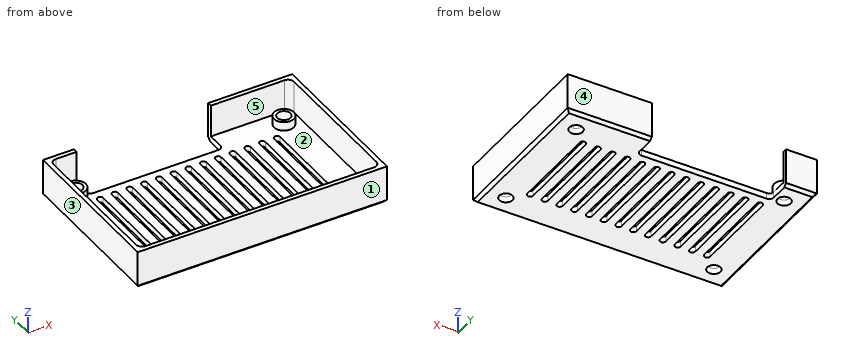
```python
from build123d import *

# Parameters (mm, degrees)
F0_W      = 84.5
F0_H      = 54
F1_DEPTH  = 11
F2_W      = 84.5
F2_H      = 54
F3_DEPTH  = 2
F4_R      = 2.25
F5_DEPTH  = 12.5
F6_R      = 3.35
F6_R_2    = 2.25
F7_DEPTH  = 3
F8_SIZE   = 1
F10_DEPTH = 2


with BuildPart() as f1:
    # F0 (on Top) → F1 (new body)
    with BuildSketch(Plane.XY):
        Rectangle(F0_W, F0_H)
        with BuildLine():
            Line((-40.75, -23.5), (-40.75, 23.5))
            ThreePointArc((-40.75, 23.5), (-40.164214, 24.914214), (-38.75, 25.5))
            Line((-38.75, 25.5), (38.75, 25.5))
            ThreePointArc((38.75, 25.5), (40.164214, 24.914214), (40.75, 23.5))
            Line((40.75, 23.5), (40.75, -23.5))
            ThreePointArc((40.75, -23.5), (40.164214, -24.914214), (38.75, -25.5))
            Line((38.75, -25.5), (-38.75, -25.5))
            ThreePointArc((-38.75, -25.5), (-40.164214, -24.914214), (-40.75, -23.5))
        make_face(mode=Mode.SUBTRACT)
    extrude(amount=F1_DEPTH)

    # F2 (on face) → F3 (join)
    with BuildSketch(Plane(origin=(0, 0, 0), x_dir=(1, 0, 0), z_dir=(0, 0, -1))):
        Rectangle(F2_W, F2_H)
    extrude(amount=F3_DEPTH)

    # F4 (on face) → F5 (cut, symmetric)
    with BuildSketch(Plane.XY):
        with Locations((-35.25, 20)):
            Circle(F4_R)
        with BuildLine():
            ThreePointArc((-31.75, 20), (-31.31066, 18.93934), (-30.25, 18.5))
            Line((-30.25, 18.5), (12.25, 18.5))
            ThreePointArc((12.25, 18.5), (13.31066, 18.93934), (13.75, 20))
            Line((13.75, 20), (13.75, 27))
            Line((13.75, 27), (-31.75, 27))
            Line((-31.75, 27), (-31.75, 20))
        make_face()
        with Locations((-35.25, -20)):
            Circle(F4_R)
        with Locations((35.25, 20)):
            Circle(F4_R)
        with Locations((35.25, -20)):
            Circle(F4_R)
    extrude(amount=F5_DEPTH, both=True, mode=Mode.SUBTRACT)

    # F6 (on face) → F7 (join)
    with BuildSketch(Plane.XY):
        with Locations((-35.25, 20)):
            Circle(F6_R)
        with Locations((-35.25, 20)):
            Circle(F6_R_2, mode=Mode.SUBTRACT)
        with Locations((35.25, 20)):
            Circle(F6_R)
        with Locations((35.25, 20)):
            Circle(F6_R_2, mode=Mode.SUBTRACT)
        with Locations((-35.25, -20)):
            Circle(F6_R)
        with Locations((-35.25, -20)):
            Circle(F6_R_2, mode=Mode.SUBTRACT)
        with Locations((35.25, -20)):
            Circle(F6_R)
        with Locations((35.25, -20)):
            Circle(F6_R_2, mode=Mode.SUBTRACT)
    extrude(amount=F7_DEPTH)

    # F8
    f8_edges = [f1.edges().sort_by_distance(p)[0] for p in [
        (-42.25, 0, -2),
        (-37, 27, -2),
        (28, 27, -2),
        (0, -27, -2),
        (42.25, 0, -2),
    ]]
    chamfer(f8_edges, length=F8_SIZE)

    # F9 (on face) → F10 (cut, through all)
    with BuildSketch(Plane.XY):
        with BuildLine():
            ThreePointArc((1, 15), (0, 16), (-1, 15))
            Line((-1, 15), (-1, -15))
            ThreePointArc((-1, -15), (0, -16), (1, -15))
            Line((1, -15), (1, 15))
        make_face()
        with BuildLine():
            Line((6, -15), (6, 15))
            ThreePointArc((6, 15), (5, 16), (4, 15))
            Line((4, 15), (4, -15))
            ThreePointArc((4, -15), (5, -16), (6, -15))
        make_face()
        with BuildLine():
            Line((11, -15), (11, 15))
            ThreePointArc((11, 15), (10, 16), (9, 15))
            Line((9, 15), (9, -15))
            ThreePointArc((9, -15), (10, -16), (11, -15))
        make_face()
        with BuildLine():
            Line((16, -15), (16, 15))
            ThreePointArc((16, 15), (15, 16), (14, 15))
            Line((14, 15), (14, -15))
            ThreePointArc((14, -15), (15, -16), (16, -15))
        make_face()
        with BuildLine():
            Line((21, -15), (21, 15))
            ThreePointArc((21, 15), (20, 16), (19, 15))
            Line((19, 15), (19, -15))
            ThreePointArc((19, -15), (20, -16), (21, -15))
        make_face()
        with BuildLine():
            Line((26, -15), (26, 15))
            ThreePointArc((26, 15), (25, 16), (24, 15))
            Line((24, 15), (24, -15))
            ThreePointArc((24, -15), (25, -16), (26, -15))
        make_face()
        with BuildLine():
            Line((-4, -15), (-4, 15))
            ThreePointArc((-4, 15), (-5, 16), (-6, 15))
            Line((-6, 15), (-6, -15))
            ThreePointArc((-6, -15), (-5, -16), (-4, -15))
        make_face()
        with BuildLine():
            Line((-9, -15), (-9, 15))
            ThreePointArc((-9, 15), (-10, 16), (-11, 15))
            Line((-11, 15), (-11, -15))
            ThreePointArc((-11, -15), (-10, -16), (-9, -15))
        make_face()
        with BuildLine():
            Line((-14, -15), (-14, 15))
            ThreePointArc((-14, 15), (-15, 16), (-16, 15))
            Line((-16, 15), (-16, -15))
            ThreePointArc((-16, -15), (-15, -16), (-14, -15))
        make_face()
        with BuildLine():
            Line((-19, -15), (-19, 15))
            ThreePointArc((-19, 15), (-20, 16), (-21, 15))
            Line((-21, 15), (-21, -15))
            ThreePointArc((-21, -15), (-20, -16), (-19, -15))
        make_face()
        with BuildLine():
            Line((-24, -15), (-24, 15))
            ThreePointArc((-24, 15), (-25, 16), (-26, 15))
            Line((-26, 15), (-26, -15))
            ThreePointArc((-26, -15), (-25, -16), (-24, -15))
        make_face()
        with BuildLine():
            Line((-29, -15), (-29, 15))
            ThreePointArc((-29, 15), (-30, 16), (-31, 15))
            Line((-31, 15), (-31, -15))
            ThreePointArc((-31, -15), (-30, -16), (-29, -15))
        make_face()
        with BuildLine():
            Line((31, -15), (31, 15))
            ThreePointArc((31, 15), (30, 16), (29, 15))
            Line((29, 15), (29, -15))
            ThreePointArc((29, -15), (30, -16), (31, -15))
        make_face()
    extrude(amount=-F10_DEPTH, mode=Mode.SUBTRACT)


solid = f1.part
```
For this review, take the finished solid that the model builds, in its own axes (mm). Face numbers are marked on the shaded views. A direction names the side the tool comes from. Coordinates: 2 decimals unless noted, no trailing zeros. Write each loop counter-clockwise with the first axis right and the second up, starting at its lowest first coordinate (ties: lowest second). Pieces come first, ordered by that corner, then holes. Notation, with made-up numbers: (5, -28) - (58, -28) arc R24 cw to (58, -6) - close; hole circle Ø9 at (-28, 86.5). An arc over 180 degrees is marked (long way). Answer in a Markdown table with one row per item. Add a question column.
Q1. Tool access review of the marked faces 4 and 5: name each direction out of +Z, -Z, +X, -X, +Y, -Y from which nothing blocks a thin tool from reaching the whole face with its end or side.
Q2. For probe 1 along Y at (x, z) = (-35.25, -0.8); probe 2 along Y at (x, z) = (-35.25, 0.9); probe 3 along Y at (x, z) = (35.25, -1.2), list the stretches that pass through material, from the lowest coordinate up.
Q3. We need section C-C, the plane y = 3. Count the separate pieces of the cut face and the enclosed holes in it, and give its area (3 significant figures).
Q4. Draft analysis for pull direction Y (two halves, no side actions). For the marked faces 1, 2 and 3, state which applies: +Y half, -Y half, draft (parallel to the pull), parting line (faces both ways), or undercut.
Q5. We need section A-A, the plane x = -35.25. State the section outline as (y, z) points, and give its area (3 significant figures).
Q6. We need section B-B, the plane x = 0. State the section outline as (y, z) points, and give its area (3 significant figures).
Q7. We need section D-D, the plane z = 9.75. State the section outline as (x, y) points, and give its area (3 significant figures).
Q8. For P1, Ø3.5, axis at x = 6.5, z = 5, coming from the +Y side; P2, Ø8, axis at x = 33.5, y = -4, coming from the +Z side; P3, Ø1, axis at x = -16.5, z = -0.5, coming from the +Y side; P4, Ø2.5, axis at x = -35.25, y = -20, coming from the -Z side, all flat-tipped, find the tip position at first contact; note any pin that passes through.
Answer list:
| question | item | result |
|---|---|---|
| 1 | face 4 | +Z, -Z, +X, -X, +Y |
| 1 | face 5 | +Z |
| 2 | probe 1 | y = -27 to -22.25, -17.75 to 17.75, 22.25 to 27 |
| 2 | probe 2 | y = -27 to -25.5, -23.35 to -22.25, -17.75 to -16.65, 16.65 to 17.75, 22.25 to 23.35, 25.5 to 27 |
| 2 | probe 3 | y = -26.8 to -22.25, -17.75 to 17.75, 22.25 to 26.8 |
| 3 | separate pieces | 14 |
| 3 | enclosed holes | 0 |
| 3 | area | 149 mm2 |
| 4 | face 1 | -Y half |
| 4 | face 2 | undercut |
| 4 | face 3 | draft |
| 5 | outline | (-27, -1) - (-26, -2) - (-22.25, -2) - (-22.25, 3) - (-23.35, 3) - (-23.35, 0) - (-25.5, 0) - (-25.5, 11) - (-27, 11) - close; (-17.75, -2) - (17.75, -2) - (17.75, 3) - (16.65, 3) - (16.65, 0) - (-16.65, 0) - (-16.65, 3) - (-17.75, 3) - close; (22.25, -2) - (26, -2) - (27, -1) - (27, 11) - (25.5, 11) - (25.5, 0) - (23.35, 0) - (23.35, 3) - (22.25, 3) - close |
| 5 | area | 135 mm2 |
| 6 | outline | (-27, -1) - (-26, -2) - (-16, -2) - (-16, 0) - (-25.5, 0) - (-25.5, 11) - (-27, 11) - close; (16, -2) - (18.5, -2) - (18.5, 0) - (16, 0) - close |
| 6 | area | 43.0 mm2 |
| 7 | outline | (-42.25, -27) - (42.25, -27) - (42.25, 27) - (13.75, 27) - (13.75, 25.5) - (38.75, 25.5) arc R2 cw to (40.75, 23.5) - (40.75, -23.5) arc R2 cw to (38.75, -25.5) - (-38.75, -25.5) arc R2 cw to (-40.75, -23.5) - (-40.75, 23.5) arc R2 cw to (-38.75, 25.5) - (-31.75, 25.5) - (-31.75, 27) - (-42.25, 27) - close |
| 7 | area | 342 mm2 |
| 8 | P1 | stops at y = -25.5 |
| 8 | P2 | stops at z = 0 |
| 8 | P3 | stops at y = 18.5 |
| 8 | P4 | passes through |
